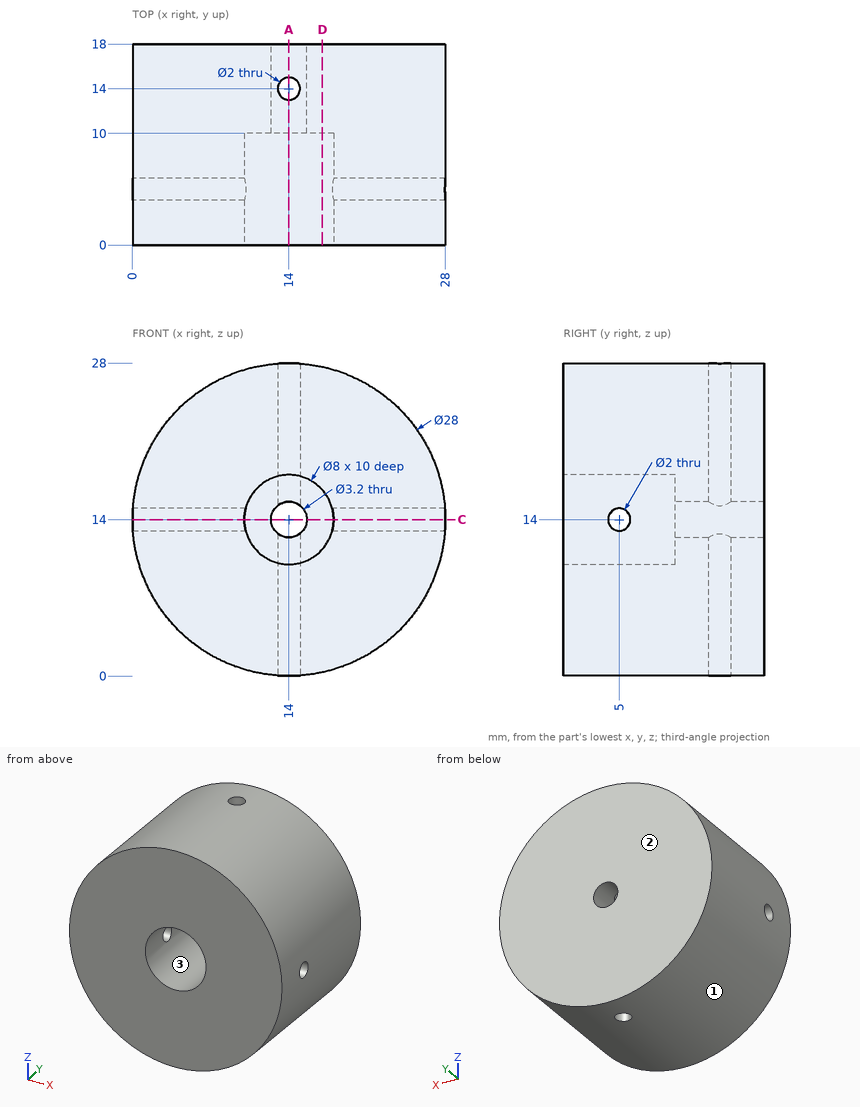
Design review of the part shown in the three views and the two pictorial views. Dimensions are in mm from the part's minimum x, y and z. Give positions to 0.01 mm unless a question says otherwise; leave off trailing zeros. Write each loop counter-clockwise with the first axis right and the second up, starting at its lowest first coordinate (ties: lowest second). Pieces come first, ordered by that corner, then holes. Notation, with made-up numbers: (77, -7) -> (90, -7) arc R9 ccw to (90, 2) -> close; hole circle Ø8 at (88.5, -31.5). An arc over 180 degrees is marked (long way). Answer in a Markdown table with one row per item.
1) Add section D-D on x = 17. State the section outline as (y, z) points, plus the area to 3 significant figures.
Worked answers:
| item | result |
|---|---|
| outline | (0, 0.33) -> (18, 0.33) -> (18, 27.67) -> (0, 27.67) -> (0, 16.65) -> (10, 16.65) -> (10, 11.35) -> (0, 11.35) -> close |
| area | 439 mm² |
2) Clearance check with flat-ended pins moving along their axes: P1, Ø10, axis at x = 15, y = 3.5, coming from the +Z side; P2, Ø1.5, axis at y = 8.5, z = 12.5, coming from the +X side; P3, Ø1.6, axis at y = 5, z = 14, coming from the +X side; P4, Ø3.5, axis at x = 14, z = 14, coming from the -Y side. State where each tip first meets the part, or that it passes through.
Worked answers:
| item | result |
|---|---|
| P1 | z = 28 |
| P2 | x = 27.98 |
| P3 | through |
| P4 | y = 10 |
3) Mouldability with a two-part tool opening along X and no side actions: class the marked faces 1, 2 and 3 as +X half, -X half, draft (parallel to the pull), parting line (faces both ways), or undercut.
Worked answers:
| item | result |
|---|---|
| face 1 | parting line |
| face 2 | draft |
| face 3 | undercut |
4) For L1, parallel to Y at x = 6, z = 14; L2, parallel to X at y = 16, z = 14; L3, parallel to X at y = 1, z = 16.25, list the stretches that pass through material, from the lowest coordinate up. Write a range as [from, to].
Worked answers:
| item | result |
|---|---|
| L1 | [0, 4], [6, 18] |
| L2 | [0, 12.4], [15.6, 28] |
| L3 | [0.18, 10.69], [17.31, 27.82] |
5) Add section A-A on x = 14. State the section outline as (y, z) points, plus the area to 3 significant figures.
Worked answers:
| item | result |
|---|---|
| outline | (0, 0) -> (13, 0) -> (13, 12.4) -> (10, 12.4) -> (10, 10) -> (0, 10) -> close; (0, 18) -> (10, 18) -> (10, 15.6) -> (13, 15.6) -> (13, 28) -> (0, 28) -> close; (15, 0) -> (18, 0) -> (18, 12.4) -> (15, 12.4) -> close; (15, 15.6) -> (18, 15.6) -> (18, 28) -> (15, 28) -> close |
| area | 349 mm² |
6) Add section C-C on z = 14. State the section outline as (x, y) points, plus the area to 3 significant figures.
Worked answers:
| item | result |
|---|---|
| outline | (0, 0) -> (10, 0) -> (10, 4) -> (0, 4) -> close; (0, 6) -> (10, 6) -> (10, 10) -> (12.4, 10) -> (12.4, 18) -> (0, 18) -> close; (15.6, 10) -> (18, 10) -> (18, 6) -> (28, 6) -> (28, 18) -> (15.6, 18) -> close; (18, 0) -> (28, 0) -> (28, 4) -> (18, 4) -> close |
| area | 358 mm² |
